The listing builds one solid part. Answer for the finished solid, in the listing's coordinates (mm). Face numbers are marked on the shaded views. Give positions to 0.01 mm unless a question says otherwise; leave off trailing zeros. Write each loop counter-clockwise with the first axis right and the second up, starting at its lowest first coordinate (ties: lowest second). Pieces come first, ordered by that corner, then holes. Notation, with made-up numbers: M -9.75,-21 L 11.25,-21 A24 ccw 11.25,10 Z; hole C 40.5,-6.75 d5. An arc over 180 degrees is marked long. Answer as a JSON object with one key per item and string values.
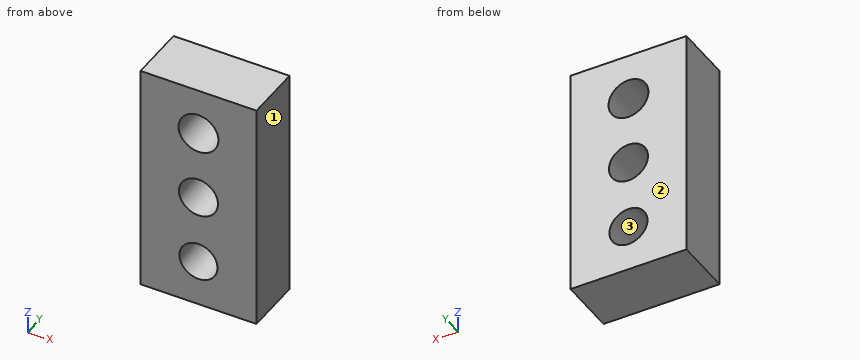
```python
from build123d import *

# Parameters (mm, degrees)
SKETCH1_W                   = 12.7
SKETCH1_H                   = 25.4
BOSS_EXTRUDE1_DEPTH         = 6.35
F_1_0_MM_DOWEL_HOLES1_D     = 4.17
F_1_0_MM_DOWEL_HOLES1_DEPTH = 7.874
F_1_0_MM_DOWEL_HOLES1_TIP   = 1.252794391
F_1_0_MM_DOWEL_HOLES2_D     = 4.27
F_1_0_MM_DOWEL_HOLES2_DEPTH = 7.874
F_1_0_MM_DOWEL_HOLES2_TIP   = 1.282837422
F_1_0_MM_DOWEL_HOLES3_D     = 4.37
F_1_0_MM_DOWEL_HOLES3_DEPTH = 7.874
F_1_0_MM_DOWEL_HOLES3_TIP   = 1.312880453


with BuildPart() as part:
    # Sketch1 → Boss-Extrude1 (new body)
    with BuildSketch(Plane(origin=(0, 0, 0), x_dir=(1, 0, 0), z_dir=(0, 1, 0))):
        Rectangle(SKETCH1_W, SKETCH1_H)
    extrude(amount=BOSS_EXTRUDE1_DEPTH)

    # Ø1.0 mm Dowel Holes1
    with Locations(Plane(origin=(0, 6.35, 0), x_dir=(1, 0, 0), z_dir=(0, 1, 0))):
        with Locations((0, 7.62)):
            Hole(F_1_0_MM_DOWEL_HOLES1_D / 2, depth=F_1_0_MM_DOWEL_HOLES1_DEPTH)
            with Locations((0, 0, -(F_1_0_MM_DOWEL_HOLES1_DEPTH + F_1_0_MM_DOWEL_HOLES1_TIP / 2))):  # 118° drill point
                Cone(0, F_1_0_MM_DOWEL_HOLES1_D / 2, F_1_0_MM_DOWEL_HOLES1_TIP, mode=Mode.SUBTRACT)

    # Ø1.0 mm Dowel Holes2
    with Locations(Plane(origin=(0, 6.35, 0), x_dir=(1, 0, 0), z_dir=(0, 1, 0))):
        with Locations((0, 0)):
            Hole(F_1_0_MM_DOWEL_HOLES2_D / 2, depth=F_1_0_MM_DOWEL_HOLES2_DEPTH)
            with Locations((0, 0, -(F_1_0_MM_DOWEL_HOLES2_DEPTH + F_1_0_MM_DOWEL_HOLES2_TIP / 2))):  # 118° drill point
                Cone(0, F_1_0_MM_DOWEL_HOLES2_D / 2, F_1_0_MM_DOWEL_HOLES2_TIP, mode=Mode.SUBTRACT)

    # Ø1.0 mm Dowel Holes3
    with Locations(Plane(origin=(0, 6.35, 0), x_dir=(1, 0, 0), z_dir=(0, 1, 0))):
        with Locations((0, -7.62)):
            Hole(F_1_0_MM_DOWEL_HOLES3_D / 2, depth=F_1_0_MM_DOWEL_HOLES3_DEPTH)
            with Locations((0, 0, -(F_1_0_MM_DOWEL_HOLES3_DEPTH + F_1_0_MM_DOWEL_HOLES3_TIP / 2))):  # 118° drill point
                Cone(0, F_1_0_MM_DOWEL_HOLES3_D / 2, F_1_0_MM_DOWEL_HOLES3_TIP, mode=Mode.SUBTRACT)


solid = part.part
```
1. The mould has two halves that part along X. Classify the marked faces 1, 2 and 3: released by +X, released by -X, zero draft, split by the parting line, or undercut.
Verdict:
{"face 1": "released by +X", "face 2": "zero draft", "face 3": "undercut"}
2. A cutting plane is placed at A-A, the plane x = 0. Give the vertices of the cut face in (y, z) (3 decimals), plus the area to 3 significant figures.
Verdict:
{"outline": "M 0,-12.7 L 6.35,-12.7 L 6.35,-9.705 L 0,-9.705 Z; M 0,-5.535 L 6.35,-5.535 L 6.35,-2.135 L 0,-2.135 Z; M 0,2.135 L 6.35,2.135 L 6.35,5.435 L 0,5.435 Z; M 0,9.805 L 6.35,9.805 L 6.35,12.7 L 0,12.7 Z", "area": "79.9 mm2"}
3. A cutting plane is placed at D-D, the plane z = 0. Give the vertices of the cut face in (x, y) (3 decimals).
Verdict:
{"outline": "M -6.35,0 L -2.135,0 L -2.135,6.35 L -6.35,6.35 Z; M 2.135,0 L 6.35,0 L 6.35,6.35 L 2.135,6.35 Z"}
4. Consider line 1 along Z through (x, y) = (0, 2.75) (3 decimals); line 2 along Z through (x, y) = (0.25, 2.5); line 3 along X through (y, z) = (4, -0.25). Determine where each line is inside the solid, lowest interval first.
Verdict:
{"line 1": "z = -12.7 to -9.705, -5.535 to -2.135, 2.135 to 5.435, 9.805 to 12.7", "line 2": "z = -12.7 to -9.69, -5.55 to -2.12, 2.12 to 5.45, 9.79 to 12.7", "line 3": "x = -6.35 to -2.12, 2.12 to 6.35"}
5. A cutting plane is placed at B-B, the plane z = 7.62. Give the vertices of the cut face in (x, y) (3 decimals).
Verdict:
{"outline": "M -6.35,0 L -2.185,0 L -2.185,6.35 L -6.35,6.35 Z; M 2.185,0 L 6.35,0 L 6.35,6.35 L 2.185,6.35 Z"}
6. A cutting plane is placed at C-C, the plane y = 1. Give the vertices of the cut face in (x, z) (3 decimals).
Verdict:
{"outline": "M -6.35,-12.7 L 6.35,-12.7 L 6.35,12.7 L -6.35,12.7 Z; hole C 0,7.62 d4.37; hole C 0,0 d4.27; hole C 0,-7.62 d4.17"}
